CAD build for the part. Positions are in the model's coordinates, mm. Round coordinates to 2 decimals unless told otherwise and drop trailing zeros. Write each loop counter-clockwise with the first axis right and the second up, starting at its lowest first coordinate (ties: lowest second). Pieces come first, ordered by that corner, then holes. Notation, with made-up numbers: (66.25, 23.25) - (84.25, 23.25) arc R19 cw to (84.25, 32.25) - close; hole circle Ø6 at (87.5, -8). An arc over 180 degrees is marked (long way). Use one line per item in the form item = value. Start each with the question number.
Item 1: Drill centre lines: L1, parallel to X at y = -6, z = -11.5; L2, parallel to X at y = 15, z = -5.5; L3, parallel to Z at x = 27.5, y = -12.5. Where is each one in solid material? Low to high.
Item 2: Pin check, flat tips, straight feed: pin 1 (4 mm diameter, centred on x = 39, y = -12.5, fed in from +Z); pin 2 (3 mm diameter, centred on x = 43, y = -10, fed in from +Z). Stop position of each tip, or through.
Item 3: Band-saw the part on B-B, the plane x = 47. List the corners of the cut face in (y, z), and give its area (3 significant figures).
Item 4: Band-saw the part on A-A, the plane y = -11.5. List the corners of the cut face in (x, z), and give its area (3 significant figures).
Autodesk Inventor part; units mm, degrees
ref_plane "工作平面1" through (10, 19, 0) normal (-0.3499, -0.6624, -0.6624) x (0.8842, 0, -0.4671)
ref_plane "YZ Plane" through (0, 0, 0) normal (1, 0, 0) x (0, 1, 0)
ref_plane "XZ Plane" through (0, 0, 0) normal (0, 1, 0) x (-1, 0, 0)
sketch "草圖1" plane through (0, 0, 0) normal (0, 1, 0) x (-1, 0, 0)
  line L0 (0, 0) -> (-63, 0)
  line L1 (-63, 0) -> (-63, -38)
  line L2 (-63, -38) -> (0, -38)
  line L3 (0, -38) -> (0, 0)
  dimension "d0" = 63
  dimension "d1" = 38
extrude "擠出1" add sketch "草圖1" along normal mid plane 38
sketch "草圖2" plane through (0, 19, 0) normal (0, 1, 0) x (1, 0, 0)
  line L0 (0, 0) -> (63, 0)
  line L1 (10, 0) -> (63, 8)
  line L2 (63, 0) -> (63, 38)
  dimension "d4" = 10
  dimension "d5" = 30
extrude "擠出2" cut sketch "草圖2" against normal blind 40
sketch "草圖3" plane through (63, -19, -38) normal (1, 0, 0) x (0, 0, -1)
  line L0 (-30, 18) -> (-10, 38)
  line L1 (0, 38) -> (-38, 38)
  line L2 (-30, 38) -> (-30, 0)
  point P0 (-38, 19)
  dimension "d8" = 20
  dimension "d9" = 20
ref_plane "工作平面1" through (10, 19, 0) normal (-0.3499, -0.6624, -0.6624) x (0.8842, 0, -0.4671)
sketch "草圖4" plane through (10, 19, 0) normal (-0.3499, -0.6624, -0.6624) x (0.8842, 0, -0.4671)
  line L0 (-15.1543, -12.3218) -> (93.717, -12.3218)
  line L1 (93.717, -12.3218) -> (93.717, 28.8166)
  line L2 (93.717, 28.8166) -> (-15.1543, 28.8166)
  line L3 (-15.1543, 28.8166) -> (-15.1543, -12.3218)
  point P0 (-8.8419, 11.1397)
extrude "擠出3" cut sketch "草圖4" against normal blind 40
mirror "鏡射1" about plane through (0, 0, 0) normal (0, 1, 0) of "擠出3"
properties part number "29"
Determined:
q1.L1 = 0 to 56.38
q1.L2 = 0 to 27.98
q1.L3 = -38 to -2.75
q2.pin_1 = -6.56
q2.pin_2 = -6.74
q3.outline = (-19, -38) - (19, -38) - (19, -19.55) - (5.04, -5.58) - (-5.04, -5.58) - (-19, -19.55) - close
q3.area = 1,040 mm²
q4.outline = (0, -38) - (63, -38) - (63, -20.5) - (29.87, -3) - (10, 0) - (0, 0) - close
q4.area = 1,970 mm²
